Can you work these out from the drawing? Everything is in mm from the part's minimum corner. Round coordinates to 2 decimals unless told otherwise and drop trailing zeros. Write each loop counter-clockwise with the first axis right and the second up, starting at its lowest first coordinate (ties: lowest second). Pieces come first, ordered by that corner, then holes. Notation, with made-up numbers: (22.25, 7) - (81.25, 7) arc R12 cw to (81.25, 22) - close; hole circle Ø8 at (-20, -1.75). An arc over 180 degrees is marked (long way). One line per item, written item: value. Start each with the question number.
(1) I'm going to push flat-ended pins straight in: pin 1 Ø1 at (x, z) = (67, 56) entering from +Y; pin 2 Ø10 at (x, y) = (67, 27.5) entering from +Z; pin 3 Ø16 at (x, y) = (34.5, 25.5) entering from +Z. Where does each tip first touch, or does it pass through?
(2) I want a section at D-D on x = 30. List the corners of the cut face in (y, z) for me.
(3) I want a section at B-B on y = 30. List the corners of the cut face in (x, z) for me, plus the area to 3 significant figures.
(4) If I drill on L1, parallel to Y at x = 70, z = 19.5; L2, parallel to Z at x = 123.5, y = 7; L3, parallel to X at y = 31, z = 30, over which ranges is the centre line in solid material (lowest first)? Write a range as from..to.
(5) Thinking about a two-plate mould opening in X: for the marked faces 1, 2 and 3, which applies, +X half, -X half, draft (parallel to the pull), parting line (faces both ways), or undercut?
(6) I want a section at A-A on x = 70. List the corners of the cut face in (y, z) for me, plus the area to 3 significant figures.
(7) I want a section at C-C on z = 8.5. List the corners of the cut face in (x, y) for me.
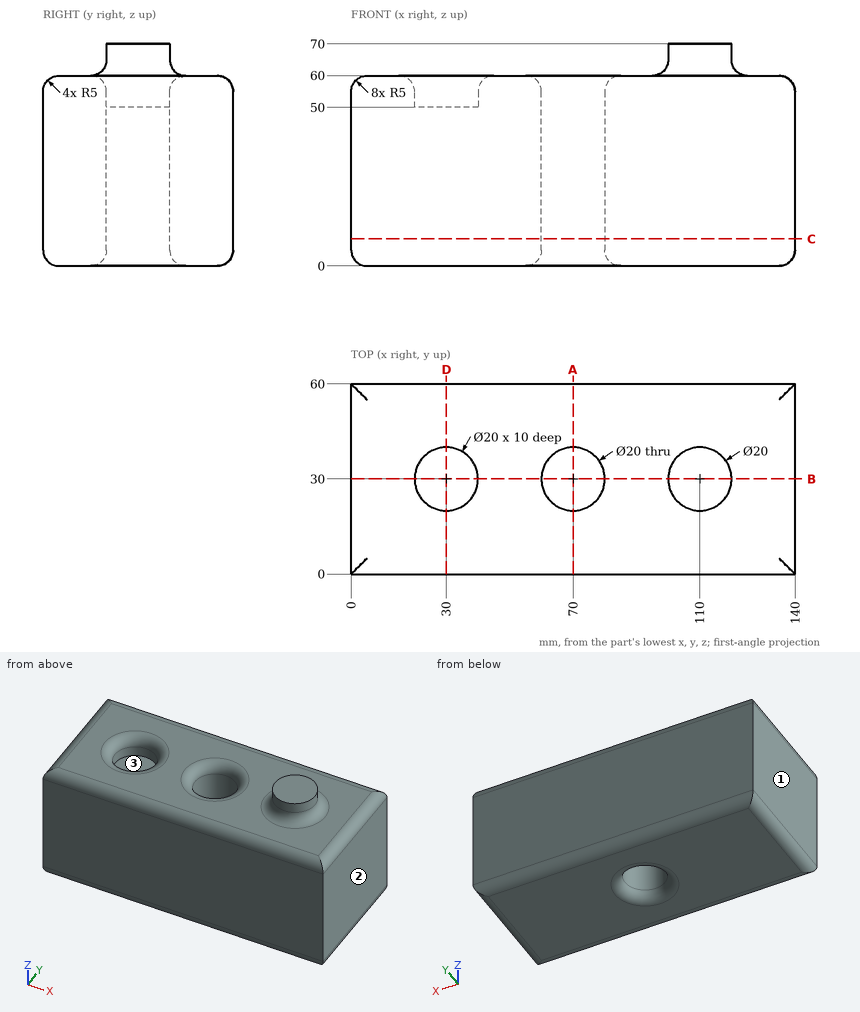
Established:
1. pin 1: y = 59.97
1. pin 2: through
1. pin 3: z = 59.96
2. outline: (0, 5) arc R5 ccw to (5, 0) - (55, 0) arc R5 ccw to (60, 5) - (60, 55) arc R5 ccw to (55, 60) - (45, 60) arc R5 ccw to (40, 55) - (40, 50) - (20, 50) - (20, 55) arc R5 ccw to (15, 60) - (5, 60) arc R5 ccw to (0, 55) - close
3. outline: (0, 5) arc R5 ccw to (5, 0) - (55, 0) arc R5 ccw to (60, 5) - (60, 55) arc R5 ccw to (55, 60) - (45, 60) arc R5 ccw to (40, 55) - (40, 50) - (20, 50) - (20, 55) arc R5 ccw to (15, 60) - (5, 60) arc R5 ccw to (0, 55) - close; (80, 5) arc R5 ccw to (85, 0) - (135, 0) arc R5 ccw to (140, 5) - (140, 55) arc R5 ccw to (135, 60) - (125, 60) arc R5 cw to (120, 65) - (120, 70) - (100, 70) - (100, 65) arc R5 cw to (95, 60) - (85, 60) arc R5 ccw to (80, 55) - close
3. area: 7,160 mm2
4. L1: 0..20, 40..60
4. L2: 0..60
4. L3: 0..60.05, 79.95..140
5. face 1: -X half
5. face 2: +X half
5. face 3: undercut
6. outline: (0, 5) arc R5 ccw to (5, 0) - (15, 0) arc R5 ccw to (20, 5) - (20, 55) arc R5 ccw to (15, 60) - (5, 60) arc R5 ccw to (0, 55) - close; (40, 5) arc R5 ccw to (45, 0) - (55, 0) arc R5 ccw to (60, 5) - (60, 55) arc R5 ccw to (55, 60) - (45, 60) arc R5 ccw to (40, 55) - close
6. area: 2,360 mm2
7. outline: (0, 0) - (140, 0) - (140, 60) - (0, 60) - close; hole circle Ø20 at (70, 30)
